For this review, take the finished solid that the model builds, in its own axes (mm). Face numbers are marked on the shaded views. A direction names the side the tool comes from. Round coordinates to 2 decimals unless told otherwise and drop trailing zeros. Loops run counter-clockwise (first coordinate to the right, second up) from the corner with the lowest first, then second, coordinate; pieces in that order, holes last.
1) Take a section at A-A (x = 0). State the section outline as (y, z) points, then the cut area to 3 significant figures.
2) Take a section at B-B (z = 4.1). State the section outline as (x, y) points.
3) Take a section at D-D (z = 2.2). State the section outline as (x, y) points, then the cut area to 3 significant figures.
4) Wall thickness on L1, parallel to Y at x = 0, z = 1.7; L2, parallel to Z at x = -2.05, y = 2.05; L3, parallel to Z at x = -2.1, y = 0.1: over which ranges is each line inside the solid? List them lowest first.
5) Insertion check: pin 1 (1 mm diameter, centred on x = 0, y = -0.5, fed in from -Z); pin 2 (1.5 mm diameter, centred on x = 1, y = -1.5, fed in from +Z); pin 3 (0.5 mm diameter, centred on y = -1, z = 4, fed in from +X). Each pin has a flat end and moves straight along its axis. Give the tip position at first contact, or say it passes through.
6) Mouldability with a two-part tool opening along X and no side actions: class the marked faces 4, 5 and 6 as pulls with the +X half, pulls with the -X half, needs draft (parallel to the pull), parting line crosses it, or undercut.
7) Tool access review of the marked faces 1, 2 and 3: name each direction out of +Z, -Z, +X, -X, +Y, -Y from which nothing blocks a thin tool from reaching the whole face with its end or side.
Autodesk Inventor part; units mm, degrees
ref_plane "作業平面1" through (0, 0, 4.5) normal (0, 0, 1) x (1, 0, 0)
ref_plane "YZ Plane" through (0, 0, 0) normal (1, 0, 0) x (0, 1, 0)
ref_plane "XZ Plane" through (0, 0, 0) normal (0, 1, 0) x (-1, 0, 0)
sketch "スケッチ1" plane through (0, 0, 0) normal (0, 0, 1) x (1, 0, 0)
  circle A0 centre (0, 0) radius 1.6
  circle A1 centre (0, 0) radius 3
  dimension "d0" = 3.2
  dimension "d1" = 6
extrude "押し出し1" add sketch "スケッチ1" along normal blind 2.5
sketch "スケッチ2" plane through (0, 0, 0) normal (1, 0, 0) x (0, 1, 0)
  arc A0 (2.85, 3.5) -> (-2.85, 3.5) centre (0, -0.0613) ccw
  line L0 (2.85, 3.5) -> (-2.85, 3.5)
  line L1 (-2.85, 3.5) -> (-2.85, 2.5)
  line L2 (-2.85, 2.5) -> (2.85, 2.5)
  line L3 (2.85, 2.5) -> (2.85, 3.5)
  line L4 (3, 2.5) -> (-3, 2.5)
  line L5 (10, 4.5) -> (-10, 4.5)
  line L6 (0, 2.5) -> (0, 4.5)
  point P0 (0, 0)
  point P1 (0, 4.5)
  dimension "d4" = 1
  dimension "d5" = 1
  dimension "d7" = 5.7
revolve "回転1" add sketch "スケッチ2" angle 360 about axis through (0, 0, 2.5) along (0, 0, 1) picked at (1.6112, 3.682) contours L0 L6 A0 | L3 L2 L6 L0
ref_plane "作業平面1" through (0, 0, 4.5) normal (0, 0, 1) x (1, 0, 0)
sketch "スケッチ3" plane through (0, 0, 4.5) normal (0, 0, 1) x (1, 0, 0)
  line L0 (2.25, -0.5) -> (-2.25, -0.5)
  line L1 (-2.25, -0.5) -> (-2.25, 0.5)
  line L2 (-2.25, 0.5) -> (2.25, 0.5)
  line L3 (2.25, 0.5) -> (2.25, -0.5)
  line L4 (2.25, -0.5) -> (-2.25, 0.5) construction
  line L5 (-2.25, -0.5) -> (2.25, 0.5) construction
  line L6 (-0.5, -2.25) -> (0.5, -2.25)
  line L7 (0.5, -2.25) -> (0.5, 2.25)
  line L8 (0.5, 2.25) -> (-0.5, 2.25)
  line L9 (-0.5, 2.25) -> (-0.5, -2.25)
  line L10 (-0.5, -2.25) -> (0.5, 2.25) construction
  line L11 (0.5, -2.25) -> (-0.5, 2.25) construction
  point P0 (0, 0)
  point P1 (-0.5, 0.5)
  point P2 (-0.5, -0.5)
  point P3 (0.5, -0.5)
  point P4 (0.5, 0.5)
  dimension "d9" = 4.5
  dimension "d10" = 1
extrude "押し出し2" cut sketch "スケッチ3" against normal blind 1
properties part number "bearing_3_6_2.5" material "アルミニウム 6061"
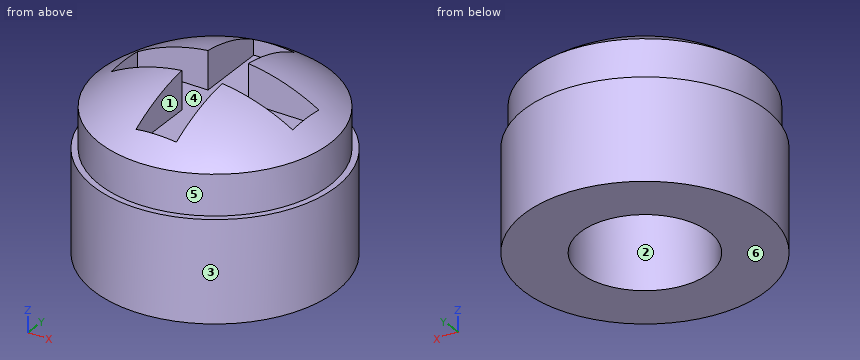
Response:
1. outline: (-3, 0) - (-1.6, 0) - (-1.6, 2.5) - (1.6, 2.5) - (1.6, 0) - (3, 0) - (3, 2.5) - (2.85, 2.5) - (2.85, 3.5) arc R4.56 ccw to (2.25, 3.91) - (2.25, 3.5) - (-2.25, 3.5) - (-2.25, 3.91) arc R4.56 ccw to (-2.85, 3.5) - (-2.85, 2.5) - (-3, 2.5) - close
1. area: 13.0 mm2
2. outline: (-1.8, -0.5) arc R1.87 ccw to (-0.5, -1.8) - (-0.5, -0.5) - close; (-1.8, 0.5) - (-0.5, 0.5) - (-0.5, 1.8) arc R1.87 ccw to start; (0.5, -1.8) arc R1.87 ccw to (1.8, -0.5) - (0.5, -0.5) - close; (0.5, 0.5) - (1.8, 0.5) arc R1.87 ccw to (0.5, 1.8) - close
3. outline: circle Ø6 at (0, 0); hole circle Ø3.2 at (0, 0)
3. area: 20.2 mm2
4. L1: y = -3 to -1.6, 1.6 to 3
4. L2: z = 0 to 2.5
4. L3: z = 0 to 3.5
5. pin 1: stops at z = 2.5
5. pin 2: stops at z = 4.38
5. pin 3: stops at x = 2.31
6. face 4: undercut
6. face 5: parting line crosses it
6. face 6: needs draft
7. face 1: +Z
7. face 2: -Z
7. face 3: +Z, -Z
